Check sheet for the modelled part. Datum: model origin and axes. Units: mm. A direction names the side the tool comes from. Round coordinates to 2 decimals unless told otherwise and drop trailing zeros. Write each loop counter-clockwise with the first axis right and the second up, starting at its lowest first coordinate (ties: lowest second). Pieces come first, ordered by that corner, then holes. Notation, with made-up numbers: M 55,-31 L 73,-31 A22 ccw 73,-19 Z; hole C 37.25,20 d8. An arc over 180 degrees is marked long. Answer in a Markdown table with one row per item.
```python
from build123d import *

# Parameters (mm, degrees)
F0_W     = 577.85
F0_H     = 355.6
F1_DEPTH = 304.8
F2_W     = 565.15
F2_H     = 292.1
F3_DEPTH = 352.425
F4_W     = 558.8
F4_H     = 141.224
F5_DEPTH = 352.425
F7_DEPTH = 25.4


with BuildPart() as f1:
    # F0 (on Top) → F1 (new body)
    with BuildSketch(Plane.XY):
        Rectangle(F0_W, F0_H)
    extrude(amount=F1_DEPTH)

    # F2 (on face) → F3 (cut)
    with BuildSketch(Plane.XZ.offset(177.8)):
        with Locations((0, 152.4)):
            Rectangle(F2_W, F2_H)
    extrude(amount=-F3_DEPTH, mode=Mode.SUBTRACT)

    # F4 (on face) → F5 (join)
    with BuildSketch(Plane.XZ.offset(-174.625)):
        with Locations((0, 224.663)):
            Rectangle(F4_W, F4_H)
        with Locations((0, 80.137)):
            Rectangle(F4_W, F4_H)
    extrude(amount=F5_DEPTH)

    # F6 (on face) → F7 (cut)
    with BuildSketch(Plane.XZ.offset(177.8)):
        with BuildLine():
            Line((101.6, 138.049), (0, 138.049))
            Line((0, 138.049), (0, 36.449))
            Line((0, 36.449), (101.6, 36.449))
            ThreePointArc((101.6, 36.449), (152.4, 87.249), (101.6, 138.049))
        make_face()
        with BuildLine():
            Line((0, 36.449), (0, 138.049))
            Line((0, 138.049), (-101.6, 138.049))
            ThreePointArc((-101.6, 138.049), (-152.4, 87.249), (-101.6, 36.449))
            Line((-101.6, 36.449), (0, 36.449))
        make_face()
        with BuildLine():
            Line((0, 282.575), (-101.6, 282.575))
            ThreePointArc((-101.6, 282.575), (-152.4, 231.775), (-101.6, 180.975))
            Line((-101.6, 180.975), (0, 180.975))
            Line((0, 180.975), (0, 282.575))
        make_face()
        with BuildLine():
            Line((101.6, 282.575), (0, 282.575))
            Line((0, 282.575), (0, 180.975))
            Line((0, 180.975), (101.6, 180.975))
            ThreePointArc((101.6, 180.975), (152.4, 231.775), (101.6, 282.575))
        make_face()
    extrude(amount=-F7_DEPTH, mode=Mode.SUBTRACT)


solid = f1.part
```
1. Draft check along X on faces 1 (the face through (288.925, -2, 150)), 2 (the face through (-4, 2, 304.8)), 3 (the face through (279.4, 1, 79)). Enter one of: +X half, -X half, draft (parallel to the pull), parting line (faces both ways), or undercut.
Found:
| item | result |
|---|---|
| face 1 | +X half |
| face 2 | draft |
| face 3 | undercut |
2. Section check B-B, the plane x = -174. Record the cut outline in (y, z) (3 decimals).
Found:
| item | result |
|---|---|
| outline | M -177.8,0 L 177.8,0 L 177.8,304.8 L -177.8,304.8 L -177.8,298.45 L 174.625,298.45 L 174.625,295.275 L -177.8,295.275 L -177.8,154.051 L 174.625,154.051 L 174.625,150.749 L -177.8,150.749 L -177.8,9.525 L 174.625,9.525 L 174.625,6.35 L -177.8,6.35 Z |
3. Access from +Z, -Z, +X, -X, +Y, -Y to the whole of each face (thin tool, end or side, straight path). Record for faces 4 (the face through (-1, -177.8, 5)), 5 (the face through (152.388, -165.278, 230.658)).
Found:
| item | result |
|---|---|
| face 4 | +Z, -Z, +X, -X, -Y |
| face 5 | -Y |
4. Go/stop test with a flat-tipped pin: pin 1 (8 mm diameter, centred on x = 100.5, z = 247.5, fed in from -Y). Record where the tip stops, or that it passes through.
Found:
| item | result |
|---|---|
| pin 1 | stops at y = -152.4 |
5. Section check D-D, the plane x = -64.5. Record the cut outline in (y, z) (3 decimals), and give its area (3 significant figures).
Found:
| item | result |
|---|---|
| outline | M -177.8,0 L 177.8,0 L 177.8,304.8 L -177.8,304.8 L -177.8,298.45 L 174.625,298.45 L 174.625,295.275 L -177.8,295.275 L -177.8,282.575 L -152.4,282.575 L -152.4,180.975 L -177.8,180.975 L -177.8,154.051 L 174.625,154.051 L 174.625,150.749 L -177.8,150.749 L -177.8,138.049 L -152.4,138.049 L -152.4,36.449 L -177.8,36.449 L -177.8,9.525 L 174.625,9.525 L 174.625,6.35 L -177.8,6.35 Z |
| area | 99,800 mm2 |
6. Section check C-C, the plane z = 68. Record the cut outline in (x, y) (3 decimals), and give its area (3 significant figures).
Found:
| item | result |
|---|---|
| outline | M -288.925,-177.8 L -282.575,-177.8 L -282.575,174.625 L -279.4,174.625 L -279.4,-177.8 L -148.612,-177.8 L -148.612,-152.4 L 148.612,-152.4 L 148.612,-177.8 L 279.4,-177.8 L 279.4,174.625 L 282.575,174.625 L 282.575,-177.8 L 288.925,-177.8 L 288.925,177.8 L -288.925,177.8 Z |
| area | 196,000 mm2 |
7. Scan lines: L1, parallel to X at y = -140.5, z = 267 (3 decimals); L2, parallel to Z at x = 113, y = -14.5 (3 decimals); L3, parallel to Y at x = 139, z = 258. Record each from-to range of solid material in increasing order.
Found:
| item | result |
|---|---|
| L1 | x = -288.925 to -282.575, -279.4 to 279.4, 282.575 to 288.925 |
| L2 | z = 0 to 6.35, 9.525 to 150.749, 154.051 to 295.275, 298.45 to 304.8 |
| L3 | y = -152.4 to 177.8 |
8. Section check A-A, the plane y = -59. Record the cut outline in (x, z) (3 decimals), and give its area (3 significant figures).
Found:
| item | result |
|---|---|
| outline | M -288.925,0 L 288.925,0 L 288.925,304.8 L -288.925,304.8 Z; M -279.4,9.525 L 279.4,9.525 L 279.4,150.749 L -279.4,150.749 Z; M -279.4,154.051 L 279.4,154.051 L 279.4,295.275 L -279.4,295.275 Z; hole M -282.575,6.35 L 282.575,6.35 L 282.575,298.45 L -282.575,298.45 Z |
| area | 169,000 mm2 |
